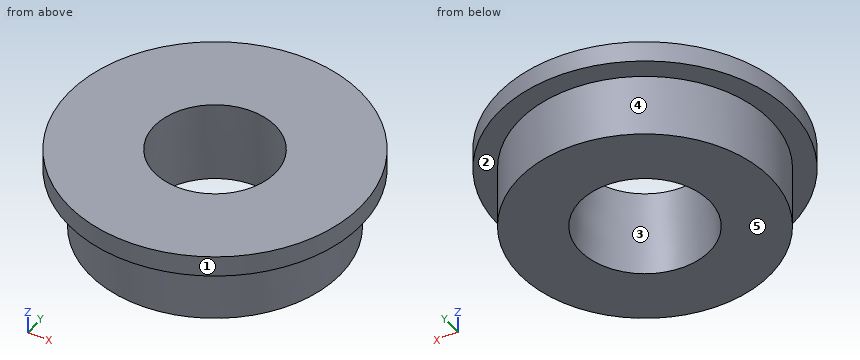
```python
from build123d import *

# Parameters (mm, degrees)
SKETCH010_R     = 14
PAD006_DEPTH    = 8
SKETCH011_R     = 14
SKETCH011_R_2   = 12
POCKET001_DEPTH = 6


with BuildPart() as part:
    # Sketch010 → Pad006 (new body)
    with BuildSketch(Plane.XY):
        Circle(SKETCH010_R)
    extrude(amount=PAD006_DEPTH)

    # Sketch011 → Pocket001 (cut)
    with BuildSketch(Plane.XY):
        Circle(SKETCH011_R)
        Circle(SKETCH011_R_2, mode=Mode.SUBTRACT)
    extrude(amount=POCKET001_DEPTH, mode=Mode.SUBTRACT)

    # Sketch012 → Groove002 (revolve, cut)
    with BuildSketch(Plane.YZ):
        Polygon((0, 0), (-6.2, 0), (-5.8, 8), (0, 8), align=None)
    revolve(axis=Axis((0, 0, 0), (0, 0, 1)), mode=Mode.SUBTRACT)


with BuildPart() as part_1:
    # Body003 placement: moved
    add(part.part.moved(Location((0, 0, -1))))


solid = part_1.part
```
Source: CAD feature listing. Evaluate the final solid. Frame: model axes, mm. Face numbers are marked on the shaded views. A direction names the side the tool comes from. Give positions to 0.01 mm unless a question says otherwise; leave off trailing zeros. Write each loop counter-clockwise with the first axis right and the second up, starting at its lowest first coordinate (ties: lowest second). Pieces come first, ordered by that corner, then holes.
1. Section query D-D (x = -10.75). Return the cut outline in (y, z).
2. Section query A-A (x = 0). Return the cut outline in (y, z).
3. Section query C-C (z = 3). Return the cut outline in (x, y), then the cut area to 3 significant figures.
4. Access query for the marked faces 1 and 2. Directions: +Z, -Z, +X, -X, +Y, -Y. A direction counts if a zero-diameter tool reaches every point of the face in a straight line with its end or side. Return the directions, or none.
5. Pull-direction query (X, two-part tool) for the marked faces 3, 4 and 5; classes: +X half, -X half, draft (parallel to the pull), parting line (faces both ways), or undercut.
6. First-contact query: pin 1 (5 mm diameter, centred on x = 11, y = 6, fed in from -Z); pin 2 (3 mm diameter, centred on y = 4.5, z = 1, fed in from -X). Flat tips, straight axial feed; report the tip coordinate or a pass-through.
7. Material intervals for line 1 along Y through (x, z) = (5.25, 2.75); line 2 along Y through (x, z) = (2.25, 0); line 3 along X through (y, z) = (-4, 6), sorted ascending.
Output values:
1. outline: (-8.97, 5) - (-5.33, 5) - (-5.33, -1) - (5.33, -1) - (5.33, 5) - (8.97, 5) - (8.97, 7) - (-8.97, 7) - close
2. outline: (-14, 5) - (-12, 5) - (-12, -1) - (-6.2, -1) - (-5.8, 7) - (-14, 7) - close; (5.8, 7) - (6.2, -1) - (12, -1) - (12, 5) - (14, 5) - (14, 7) - close
3. outline: circle Ø24 at (0, 0); hole circle Ø12 at (0, 0)
3. area: 339 mm2
4. face 1: +Z, -Z
4. face 2: -Z
5. face 3: undercut
5. face 4: parting line
5. face 5: draft
6. pin 1: stops at z = -1
6. pin 2: stops at x = -11.62
7. line 1: y = -10.79 to -2.93, 2.93 to 10.79
7. line 2: y = -11.79 to -5.72, 5.72 to 11.79
7. line 3: x = -13.42 to -4.27, 4.27 to 13.42
